The model under review builds one solid part; all positions refer to its coordinate system, in mm. Face numbers are marked on the shaded views. Coordinates: 2 decimals unless noted, no trailing zeros. Loops run counter-clockwise (first coordinate to the right, second up) from the corner with the lowest first, then second, coordinate; pieces in that order, holes last. Notation, with made-up numbers: M 54.25,10.5 L 95.25,10.5 A10 cw 95.25,25.5 Z; hole C 49,40.25 d2. An arc over 180 degrees is marked long. One line per item, written item: value.
```python
from build123d import *

# Parameters (mm, degrees)
F1_DEPTH = 19.05
F2_W     = 25.4
F2_H     = 114.3
F3_DEPTH = 361.95
F5_DEPTH = 762


with BuildPart() as f1:
    # F0 (on Front) → F1 (new body)
    with BuildSketch(Plane.XZ):
        with BuildLine():
            Line((381, 0), (-381, 0))
            Line((-381, 0), (-381, -114.3))
            Line((-381, -114.3), (-330.2, -114.3))
            Line((-330.2, -114.3), (-330.2, -88.9))
            ThreePointArc((-330.2, -88.9), (0, -63.5), (330.2, -88.9))
            Line((330.2, -88.9), (330.2, -114.3))
            Line((330.2, -114.3), (381, -114.3))
            Line((381, -114.3), (381, 0))
        make_face()
    extrude(amount=F1_DEPTH)

    # F2 (on face) → F3 (join)
    with BuildSketch(Plane(origin=(0, 0, 0), x_dir=(-1, 0, 0), z_dir=(0, 1, 0))):
        with Locations((-368.3, -57.15)):
            Rectangle(F2_W, F2_H)
        with Locations((368.3, -57.15)):
            Rectangle(F2_W, F2_H)
    extrude(amount=F3_DEPTH)

    # F4 (on face) → F5 (cut)
    with BuildSketch(Plane(origin=(-381, 0, 0), x_dir=(0, -1, 0), z_dir=(-1, 0, 0))):
        with BuildLine():
            Line((-311.15, -88.9), (-311.15, -114.3))
            Line((-311.15, -114.3), (-31.75, -114.3))
            Line((-31.75, -114.3), (-31.75, -88.9))
            ThreePointArc((-31.75, -88.9), (-171.45, -63.5), (-311.15, -88.9))
        make_face()
    extrude(amount=-F5_DEPTH, mode=Mode.SUBTRACT)


solid = f1.part
```
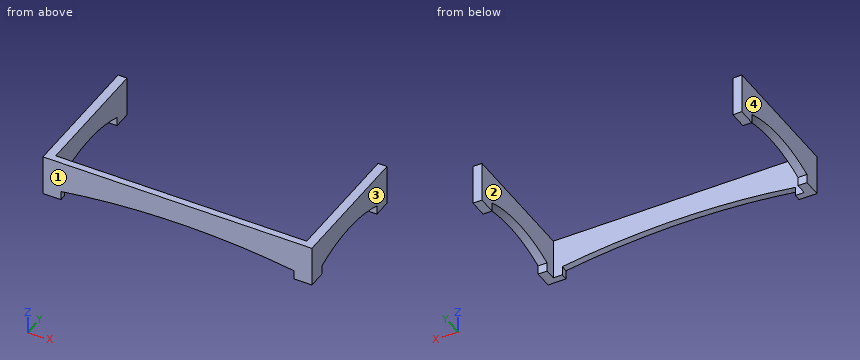
(1) Draft analysis for pull direction X (two halves, no side actions). For the marked faces 1, 2, 3 and 4, state which applies: pulls with the +X half, pulls with the -X half, needs draft (parallel to the pull), parting line crosses it, or undercut.
Checks:
face 1: needs draft
face 2: undercut
face 3: pulls with the +X half
face 4: pulls with the -X half
(2) Add section C-C on z = -80.5. State the section outline as (x, y) points, then the cut area to 3 significant figures.
Checks:
outline: M -381,-19.05 L -270.4,-19.05 L -270.4,0 L -355.6,0 L -355.6,56.54 L -381,56.54 Z; M -381,286.36 L -355.6,286.36 L -355.6,361.95 L -381,361.95 Z; M 270.4,-19.05 L 381,-19.05 L 381,56.54 L 355.6,56.54 L 355.6,0 L 270.4,0 Z; M 355.6,286.36 L 381,286.36 L 381,361.95 L 355.6,361.95 Z
area: 10,900 mm^2
(3) Insertion check: pin 1 Ø8 at (x, z) = (-179, -30.5) entering from +Y. The pin has a flat end and moves straight along its axis. Give the tip position at first contact, or say it passes through.
Checks:
pin 1: y = 0
(4) Add section A-A on y = 271.5. State the section outline as (x, z) points.
Checks:
outline: M -381,-76.32 L -355.6,-76.32 L -355.6,0 L -381,0 Z; M 355.6,-76.32 L 381,-76.32 L 381,0 L 355.6,0 Z
(5) Add section B-B on z = -14. State the section outline as (x, y) points, then the cut area to 3 significant figures.
Checks:
outline: M -381,-19.05 L 381,-19.05 L 381,361.95 L 355.6,361.95 L 355.6,0 L -355.6,0 L -355.6,361.95 L -381,361.95 Z
area: 32,900 mm^2
(6) Add section D-D on y = 47. State the section outline as (x, z) points.
Checks:
outline: M -381,-83.52 L -355.6,-83.52 L -355.6,0 L -381,0 Z; M 355.6,-83.52 L 381,-83.52 L 381,0 L 355.6,0 Z
(7) To check wall thickness, follow L1, parallel to X at y = 321, z = -68; L2, parallel to Y at x = 236, z = -52. State the ranges of each line that lie inside material, in increasing order. Write a range as [from, to].
Checks:
L1: [-381, -355.6], [355.6, 381]
L2: [-19.05, 0]
